For this review, take the finished solid that the model builds, in its own axes (mm). A direction names the side the tool comes from. Coordinates: 2 decimals unless noted, no trailing zeros. Order: outer loops, then holes, each group sorted by start corner. A loop starts at its lowest first (then second) coordinate and runs counter-clockwise, first axis right, second up. Notation, with made-up numbers: M -15.75,67.25 L -9.75,67.25 A21 cw -9.75,106.25 Z; hole C -16.75,80.25 d8. An arc over 180 degrees is marked long. Use CSV: the item, a comma, the result in double quotes.
Autodesk Inventor part; units mm, degrees
ref_plane "YZ Plane" through (0, 0, 0) normal (1, 0, 0) x (0, 1, 0)
ref_plane "XZ Plane" through (0, 0, 0) normal (0, 1, 0) x (-1, 0, 0)
ref_plane "XY Plane" through (0, 0, 0) normal (0, 0, 1) x (1, 0, 0)
sketch "Sketch1" plane through (0, 0, 0) normal (0, 0, 1) x (1, 0, 0)
  line L0 (0, -15) -> (0, 15) construction
  line L1 (-4, -15) -> (-4, 15)
  line L2 (4, 15) -> (4, -15)
  arc A0 (-4, -15) -> (0, -19) centre (0, -15) ccw
  arc A1 (4, 15) -> (-4, 15) centre (0, 15) ccw
  line L3 (4, -15) -> (0, -15)
  line L4 (-4, -11) -> (-4, -19)
  line L5 (-4, -19) -> (4, -19)
  line L6 (4, -19) -> (4, -15)
  point P0 (0, 0)
  point P1 (0, 0)
  dimension "d0" = 4
  dimension "d17" = 30
extrude "Extrusion1" add sketch "Sketch1" along normal blind 10 contours L1 A1 L2 L6 L5 A0
sketch "Sketch2" plane through (0, 0, 10) normal (0, 0, 1) x (1, 0, 0)
  line L0 (-4, 15) -> (-4, -15)
  arc A0 (-4, -15) -> (0, -19) centre (0, -15) ccw
  line L1 (4, -19) -> (4, 15)
  arc A1 (4, 15) -> (-4, 15) centre (0, 15) ccw
  circle A2 centre (0, 0) radius 13
  circle A3 centre (0, 0) radius 3.75
  line L2 (0, -19) -> (4, -19)
  dimension "d3" = 26
  dimension "d4" = 7.5
extrude "Extrusion2" cut sketch "Sketch2" against normal blind 7 contours A2 L1 L0 | L0 A2 | A2 L1
sketch "Sketch3" plane through (0, 0, 10) normal (0, 0, 1) x (1, 0, 0)
  circle A0 centre (0, 0) radius 3.75
  circle A1 centre (0, 0) radius 2
  line L0 (-4, 15) -> (-4, 12.3693)
  line L1 (4, -19) -> (4, -12.3693)
  arc A2 (4, 12.3693) -> (-4, 12.3693) centre (0, 0) ccw
  line L2 (4, 12.3693) -> (4, 15)
  arc A3 (4, 15) -> (-4, 15) centre (0, 15) ccw
  arc A4 (-4, -12.3693) -> (4, -12.3693) centre (0, 0) ccw
  line L3 (-4, -12.3693) -> (-4, -15)
  arc A5 (-4, -15) -> (0, -19) centre (0, -15) ccw
  line L4 (0, -19) -> (4, -19)
  dimension "d7" = 4
extrude "Extrusion3" cut sketch "Sketch3" against normal through all contours A1
sketch "Sketch4" plane through (0, 0, 0) normal (0, 0, -1) x (-1, 0, 0)
  circle A0 centre (0, 0) radius 2
  line L0 (4, -15) -> (4, 15)
  arc A1 (4, 15) -> (-4, 15) centre (0, 15) ccw
  line L1 (-4, 15) -> (-4, -19)
  arc A2 (0, -19) -> (4, -15) centre (0, -15) ccw
  circle A3 centre (0, 0) radius 2
  line L2 (1.5898, -2.7772) -> (-1.6102, -2.7654)
  line L3 (-1.6102, -2.7654) -> (-3.2, 0.0118)
  line L4 (-3.2, 0.0118) -> (-1.5898, 2.7772)
  line L5 (-1.5898, 2.7772) -> (1.6102, 2.7654)
  line L6 (1.6102, 2.7654) -> (3.2, -0.0118)
  line L7 (3.2, -0.0118) -> (1.5898, -2.7772)
  circle A4 centre (0, 0) radius 3.2
  line L8 (-4, -19) -> (0, -19)
  dimension "d10" = 6.4
extrude "Extrusion4" cut sketch "Sketch4" against normal blind 3 contours L2 L3 L4 L5 L6 L7
sketch "Sketch8" plane through (0, 0, 10) normal (0, 0, 1) x (1, 0, 0)
  arc A0 (4, 12.3693) -> (-4, 12.3693) centre (0, 0) ccw
  line L0 (4, 12.3693) -> (4, 15)
  arc A1 (4, 15) -> (-4, 15) centre (0, 15) ccw
  line L1 (-4, 15) -> (-4, 12.3693)
  circle A2 centre (0, 16) radius 1.65
  dimension "d28" = 3.3
extrude "Extrusion8" cut sketch "Sketch8" against normal through all contours A2
sketch "Sketch9" plane through (-4, -15, 0) normal (-1, 0, 0) x (0, 0, 1)
  line L0 (0, 0) -> (10, 0)
  line L1 (5, 0) -> (5, -2.3027) construction
  line L2 (3, 0) -> (3, -2.3027)
  line L3 (7, -2.3027) -> (7, 0)
  arc A0 (7, 0) -> (3, 0) centre (5, 0) ccw
  arc A1 (3, -2.3027) -> (7, -2.3027) centre (5, -2.3027) ccw
  line L4 (3, 2.6307) -> (3, 27.3693)
  point P0 (0, 15)
  point P1 (5, -1.1513)
  dimension "d31" = 4
  dimension "d34" = 2
extrude "Extrusion9" cut sketch "Sketch9" against normal blind 4
sketch "Sketch10" plane through (0, 0, 10) normal (0, 0, 1) x (1, 0, 0)
  circle A0 centre (0, 0) radius 2
  circle A1 centre (0, 0) radius 2
  circle A2 centre (0, 0) radius 3.75
extrude "Extrusion10" cut sketch "Sketch10" against normal blind 3
sketch "Sketch12" plane through (4, -19, 0) normal (1, 0, 0) x (0, 0, -1)
  line L0 (-3, 19.0118) -> (-1, 19.0118)
  line L1 (-1, 19.0118) -> (-1, 7.0118)
  line L2 (-1, 7.0118) -> (-3, 7.0118)
  line L3 (-3, 7.0118) -> (-3, 19.0118)
  line L4 (-1, 19.0118) -> (-1, 31.0118)
  line L5 (-1, 31.0118) -> (-3, 31.0118)
  line L6 (-3, 31.0118) -> (-3, 19.0118)
  point P0 (0, 19)
  dimension "d40" = 12
  dimension "d41" = 2
extrude "Extrusion11" add sketch "Sketch12" along normal blind 8
properties part number "rodamiento"
Item 1: Add section D-D on y = 16. State the section outline as (x, z) points, and give its area (3 significant figures).
Solutions:
outline,"M -3.87,0 L -1.65,0 L -1.65,10 L -3.87,10 Z; M 1.65,0 L 3.87,0 L 3.87,10 L 1.65,10 Z"
area,"44.5 mm^2"
Item 2: Add section B-B on z = 4.75. State the section outline as (x, y) points, and give its area (3 significant figures).
Solutions:
outline,"M -4,-13.02 L 0,-13.02 L 0,-19 L 4,-19 L 4,-12.37 A13 cw -4,-12.37 Z; M -4,12.37 A13 cw 4,12.37 L 4,15 A4 ccw -4,15 Z; C 0,0 d7.5; hole C 0,0 d4; hole C 0,16 d3.3"
area,"91.6 mm^2"
Item 3: Draft analysis for pull direction X (two halves, no side actions). For faces 4 (the face through (2, -2, 7)), 5 (the face through (2.406, 1.375, 1.479)), 6 (the face through (-3.746, 0.165, 5.028)), state which applies: released by +X, released by -X, zero draft, split by the parting line, or undercut.
Solutions:
face 4,"zero draft"
face 5,"undercut"
face 6,"split by the parting line"
Item 4: For faces 1 (the face through (-2, -13, 5)), 2 (the face through (2.39, -1.4, 1.48)), 3 (the face through (8, 0, 1)), list the 3-axis set-ups (+Z, -Z, +X, -X, +Y, -Y) from which the entire face can be reached by the end or side of a thin tool; tool diameter is ignored.
Solutions:
face 1,"-X"
face 2,"-Z"
face 3,"-Z, +X, +Y, -Y"
Item 5: Add section C-C on x = -1. State how many separate pieces and enclosed holes the cut face has, and give its area (3 significant figures).
Solutions:
separate pieces,"3"
enclosed holes,"0"
area,"147 mm^2"
Item 6: Add section A-A on z = 7.75. State the section outline as (x, y) points.
Solutions:
outline,"M -4,-15 A4 ccw 0,-19 L 4,-19 L 4,-12.37 A13 cw -4,-12.37 Z; M -4,12.37 A13 cw 4,12.37 L 4,15 A4 ccw -4,15 Z; hole C 0,16 d3.3"
Item 7: Clearance check with flat-ended pins moving along their axes: pin 1 Ø2.5 at (x, y) = (-1.5, -15.5) entering from -Z; pin 2 Ø6 at (x, y) = (3.5, 9) entering from +Z; pin 3 Ø5 at (x, y) = (0, 0) entering from +Z; pin 4 Ø9 at (x, y) = (9, 4) entering from -Z. State where each tip first meets the part, or that it passes through.
Solutions:
pin 1,"z = 0"
pin 2,"z = 3"
pin 3,"z = 7"
pin 4,"z = 1"
Item 8: To check wall thickness, follow line 1 along Y through (x, z) = (0, 2); line 2 along Y through (x, z) = (-0.75, 2.5); line 3 along Z through (x, y) = (2.5, -0.5). State the ranges of each line that lie inside material, in increasing order. Write a range as [from, to].
Solutions:
line 1,"[-19, -2.77], [2.77, 14.35], [17.65, 19]"
line 2,"[-18.93, -2.77], [2.77, 14.53], [17.47, 18.93]"
line 3,"[3, 7]"
